CAD build for the part. Positions are in the model's coordinates, mm. Face numbers are marked on the shaded views. A direction names the side the tool comes from. Coordinates: 2 decimals unless noted, no trailing zeros. Loops run counter-clockwise (first coordinate to the right, second up) from the corner with the lowest first, then second, coordinate; pieces in that order, holes last. Notation, with made-up numbers: M 16.25,38.25 L 46.25,38.25 A13 ccw 46.25,54.25 Z; hole C 39.5,7.25 d6. An arc over 180 degrees is marked long. Answer as a JSON object with one key per item and string values. Group by question number.
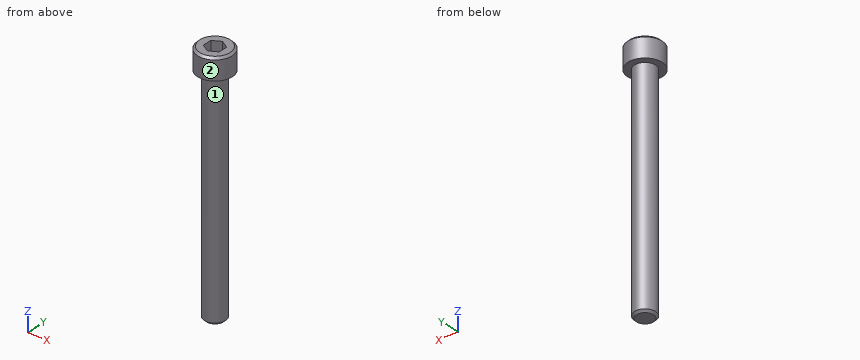
Autodesk Inventor part; units mm, degrees
ref_plane "YZ Plane" through (0, 0, 0) normal (1, 0, 0) x (0, 1, 0)
ref_plane "XZ Plane" through (0, 0, 0) normal (0, 1, 0) x (-1, 0, 0)
ref_plane "XY Plane" through (0, 0, 0) normal (0, 0, 1) x (1, 0, 0)
sketch "Sketch1" plane through (0, 0, 0) normal (0, 0, 1) x (1, 0, 0)
  circle A0 centre (0, 0) radius 4
  dimension "Diameter" = 8
extrude "Extrusion1" add sketch "Sketch1" along normal blind 85
sketch "Sketch2" plane through (0, 0, 85) normal (0, 0, 1) x (1, 0, 0)
  circle A0 centre (0, 0) radius 4
  circle A1 centre (0, 0) radius 6.5
  dimension "Head_Diameter" = 13
extrude "Extrusion2" add sketch "Sketch2" along normal blind 8 contours A0 | A1
sketch "Sketch3" plane through (0, 0, 93) normal (0, 0, 1) x (1, 0, 0)
  circle A0 centre (0, 0) radius 6.5
  circle A1 centre (0, 0) radius 3.4641 construction
  line L0 (0, 3.4641) -> (3, 1.7321)
  line L1 (3, -1.7321) -> (3, 1.7321)
  line L2 (0, 3.4641) -> (-3, 1.7321)
  line L3 (-3, -1.7321) -> (-3, 1.7321)
  line L4 (-3, -1.7321) -> (0, -3.4641)
  line L5 (3, -1.7321) -> (0, -3.4641)
  dimension "Hex_Width" = 6
extrude "Extrusion3" cut sketch "Sketch3" against normal blind 4 contours L0 L1 L5 L4 L3 L2
thread "Thread1"
chamfer "Chamfer1" distance 0.8 angle 45 2 edges at (-6.5, 0, 93) (-4, 0, 0)
equation "\"d9\" = ThreadLength"
equation "\"d12\" = Chamfer"
equation "\"ThreadLength\" = 28"
properties part number "SCREW, SOCKET HD, P, 12.9, M8X1.25X85MM"
Item 1: Slice it at A-A, the plane y = 0. Write the cut outline in (x, z), then the cut area to 3 significant figures.
Item 2: Tool access for the marked faces 1 and 2: list every direction of +Z, -Z, +X, -X, +Y, -Y with a clear straight run to the whole face (end or side of a thin tool).
Item 3: Slice it at B-B, the plane z = 60. Write the cut outline in (x, y), then the cut area to 3 significant figures.
Item 4: Pin check, flat tips, straight feed: pin 1 (2 mm diameter, centred on x = -3, z = 27, fed in from -Y); pin 2 (1 mm diameter, centred on y = -0.5, z = 46, fed in from -X); pin 3 (2 mm diameter, centred on y = 3.5, z = 74.5, fed in from +X). Stop position of each tip, or through.
Item 5: Drill centre lines: L1, parallel to X at y = -2, z = 72.5; L2, parallel to Z at x = -2.25, y = 4; L3, parallel to Z at x = -2, y = -0.5. Where is each one in solid material? Low to high. Write a range as from..to.
Computed:
{
 "1": {"outline": "M -6.5,85 L -4,85 L -4,0.8 L -3.2,0 L 3.2,0 L 4,0.8 L 4,85 L 6.5,85 L 6.5,92.2 L 5.7,93 L 3,93 L 3,89 L -3,89 L -3,93 L -5.7,93 L -6.5,92.2 Z", "area": "759 mm2"},
 "2": {"face 1": "-Z", "face 2": "+Z, -Z"},
 "3": {"outline": "C 0,0 d8", "area": "50.3 mm2"},
 "4": {"pin 1": "y = -3.46", "pin 2": "x = -4", "pin 3": "x = 3.12"},
 "5": {"L1": "-3.46..3.46", "L2": "85..93", "L3": "0..89"}
}
